from build123d import *

# Parameters (mm, degrees)
PAD_DEPTH       = 60
POCKET_DEPTH    = 61
POCKET001_DEPTH = 4.001


with BuildPart() as part:
    # Sketch001 → Pad (new body)
    with BuildSketch(Plane.XZ.offset(50)):
        with BuildLine():
            Line((0, 65), (0, 61))
            Line((0, 61), (79.226497, 61))
            ThreePointArc((79.226497, 61), (82.226497, 60.196152), (84.42265, 58))
            Line((84.42265, 58), (110.403412, 13))
            ThreePointArc((110.403412, 13), (110.403412, 7), (105.207259, 4))
            Line((105.207259, 4), (75, 4))
            Line((75, 4), (75, 0))
            Line((75, 0), (105.207259, 0))
            ThreePointArc((105.207259, 0), (113.867513, 5), (113.867513, 15))
            Line((113.867513, 15), (87.886751, 60))
            ThreePointArc((87.886751, 60), (84.226497, 63.660254), (79.226497, 65))
            Line((79.226497, 65), (0, 65))
        make_face()
    extrude(amount=-PAD_DEPTH)

    # Sketch002 (on Face12 of Pad) → Pocket (cut)
    with BuildSketch(Plane(origin=(0, -50, 65), x_dir=(-1, 0, 0), z_dir=(0, 0, 1))):
        with BuildLine():
            ThreePointArc((-70, -12), (-61.514719, -8.485281), (-58, 0))
            Line((-125.207259, 0), (-58, 0))
            Line((-125.207259, -12), (-125.207259, 0))
            Line((-70, -12), (-125.207259, -12))
        make_face()
    extrude(amount=-POCKET_DEPTH, mode=Mode.SUBTRACT)

    # Sketch003 (on Face17 of Pocket) → Pocket001 (cut, through all)
    with BuildSketch(Plane(origin=(0, -50, 4), x_dir=(-1, 0, 0), z_dir=(0, 0, 1))):
        with BuildLine():
            Line((-113.207259, 0), (-83, 0))
            ThreePointArc((-95, -12), (-86.514719, -8.485281), (-83, 0))
            Line((-95, -12), (-113.207259, -12))
            Line((-113.207259, -12), (-113.207259, 0))
        make_face()
    extrude(amount=-POCKET001_DEPTH, mode=Mode.SUBTRACT)

    # Mirrored: part across face of Pocket001


with BuildPart() as part_1:
    add(part.part)
    add(part.part.mirror(Plane(origin=(29, -50, 63), x_dir=(1, 0, 0), z_dir=(0, -1, 0))))


solid = part_1.part
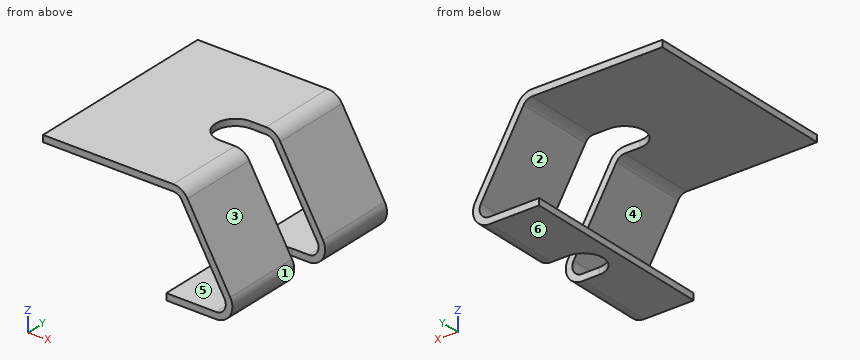
The listing builds one solid part. Answer for the finished solid, in the listing's coordinates (mm). Face numbers are marked on the shaded views. A direction names the side the tool comes from. Round coordinates to 2 decimals unless told otherwise and drop trailing zeros. Order: outer loops, then holes, each group sorted by start corner. A loop starts at its lowest first (then second) coordinate and runs counter-clockwise, first axis right, second up. Notation, with made-up numbers: M -37.75,-25 L 1.25,-25 A11 cw 1.25,-5 Z; hole C 64.25,60.5 d6. An arc over 180 degrees is marked long. Answer in a Markdown table with one row per item. Add a question column.
1) The part is cut by section C-C on z = 17. Determine the outline of the cut face in (x, y).
2) The part is cut by section A-A on x = 73.5. Determine the outline of the cut face in (y, z).
3) The part is cut by section B-B on y = -27.5. Determine the outline of the cut face in (x, z).
4) Consider line 1 along Z through (x, y) = (78, -70.5); line 2 along Z through (x, y) = (8.5, 5); line 3 along Z through (x, y) = (77.5, -44). Determine where each line is inside the solid, lowest interval first. Write a range as from..to.
5) Determine the mould class of the marked faces 3, 4, 5 and 6 for opening direction Z: pulls with the +Z half, pulls with the -Z half, needs draft (parallel to the pull), parting line crosses it, or undercut.
6) Flat-ended cylindrical pins translate along their axes: pin 1 Ø3 at (x, y) = (60.5, -11) entering from -Z; pin 2 Ø9 at (x, y) = (95.5, -73.5) entering from +Z; pin 3 Ø12 at (y, z) = (-24, 33) entering from -X. Find the tip coordinate at first contact, or state that the pin passes through.
7) The part is cut by section D-D on x = 108.5. Determine the outline of the cut face in (y, z), plus the area to 3 significant figures.
8) Which of the six approach directions +Z, -Z, +X, -X, +Y, -Y give full straight-line access (tool end or side, diameter ignored) to the marked faces 1 and 2?
Findings below:
| question | item | result |
|---|---|---|
| 1 | outline | M 108.09,-110 L 112.71,-110 L 112.71,-62 L 108.09,-62 Z; M 108.09,-38 L 112.71,-38 L 112.71,10 L 108.09,10 Z |
| 2 | outline | M -110,61 L -62,61 L -62,65 L -110,65 Z; M -38,61 L 10,61 L 10,65 L -38,65 Z |
| 3 | outline | M 0,61 L 79.23,61 A6 cw 84.42,58 L 110.4,13 A6 cw 105.21,4 L 75,4 L 75,0 L 105.21,0 A10 ccw 113.87,15 L 87.89,60 A10 ccw 79.23,65 L 0,65 Z |
| 4 | line 1 | z = 0..4, 61..65 |
| 4 | line 2 | z = 61..65 |
| 4 | line 3 | z = 0..4 |
| 5 | face 3 | pulls with the +Z half |
| 5 | face 4 | undercut |
| 5 | face 5 | undercut |
| 5 | face 6 | pulls with the -Z half |
| 6 | pin 1 | stops at z = 61 |
| 6 | pin 2 | stops at z = 54.61 |
| 6 | pin 3 | stops at x = 95.39 |
| 7 | outline | M -110,0.56 L -62,0.56 L -62,4.98 L -110,4.98 Z; M -110,16.3 L -62,16.3 L -62,24.3 L -110,24.3 Z; M -38,0.56 L 10,0.56 L 10,4.98 L -38,4.98 Z; M -38,16.3 L 10,16.3 L 10,24.3 L -38,24.3 Z |
| 7 | area | 1,190 mm² |
| 8 | face 1 | +X, +Y, -Y |
| 8 | face 2 | -X, +Y, -Y |
